Work out the finished part from the listing and answer in its coordinate system (mm). A direction names the side the tool comes from. Give positions to 0.01 mm unless a question says otherwise; leave off trailing zeros. Order: outer loops, then holes, each group sorted by start corner. A loop starts at its lowest first (then second) coordinate and runs counter-clockwise, first axis right, second up.
```python
from build123d import *

# Parameters (mm, degrees)
F1_DEPTH = 787.4
F3_DEPTH = 25.4
F4_SIZE  = 5.08


with BuildPart() as f1:
    # F0 (on Right) → F1 (new body)
    with BuildSketch(Plane.YZ):
        with BuildLine():
            Line((-17.145, 0), (0, 0))
            Line((0, 0), (0, 101.6))
            Line((0, 101.6), (-12.7, 101.6))
            Line((-12.7, 101.6), (-12.7, 98.425))
            ThreePointArc((-12.7, 98.425), (-21.680256, 94.705256), (-25.4, 85.725))
            Line((-25.4, 85.725), (-25.4, 38.1))
            Line((-25.4, 38.1), (-17.145, 38.1))
            Line((-17.145, 38.1), (-17.145, 0))
        make_face()
    extrude(amount=F1_DEPTH)

    # F2 (on face) → F3 (cut)
    with BuildSketch(Plane(origin=(0, 0, 0), x_dir=(-1, 0, 0), z_dir=(0, 1, 0))):
        Polygon((-685.8, 0), (-787.4, 101.6), (-787.4, 0), align=None)
        Polygon((0, 0), (0, 101.6), (-101.6, 0), align=None)
    extrude(amount=-F3_DEPTH, mode=Mode.SUBTRACT)

    # F4
    f4_edges = [f1.edges().sort_by_distance(p)[0] for p in [
        (393.7, -25.4, 38.1),
    ]]
    chamfer(f4_edges, length=F4_SIZE)


solid = f1.part
```
1. Which of the six approach directions +Z, -Z, +X, -X, +Y, -Y give full straight-line access (tool end or side, diameter ignored) to faces 1 (the face through (389, -17.145, 19)), 2 (the face through (50.1, -9.7, 51.5))?
Findings below:
face 1: -Z, +X, -X, -Y
face 2: -Z, -X, +Y, -Y
2. Given P1, Ø2.5, axis at x = 483.5, z = 100.5, coming from the -Y side; P2, Ø1, axis at x = 105, z = 31, coming from the -Y side (3 decimals); P3, Ø1.5, axis at x = 521, y = -22, coming from the -Z side, each flat-ended and moving along its own axis, determine where each tip first touches the part or whether it passes through.
Findings below:
P1: stops at y = -12.7
P2: stops at y = -17.145
P3: stops at z = 39.03
3. The part is cut by section A-A (x = 218). Write down the section's boundary in (y, z) (3 decimals), then the cut area to 3 significant figures.
Findings below:
outline: (-25.4, 43.18) - (-20.32, 38.1) - (-17.145, 38.1) - (-17.145, 0) - (0, 0) - (0, 101.6) - (-12.7, 101.6) - (-12.7, 98.425) arc R12.7 ccw to (-25.4, 85.725) - close
area: 2,180 mm2
4. The part is cut by section D-D (x = 700). Write down the section's boundary in (y, z) (3 decimals).
Findings below:
outline: (-25.4, 43.18) - (-20.32, 38.1) - (-17.145, 38.1) - (-17.145, 14.2) - (0, 14.2) - (0, 101.6) - (-12.7, 101.6) - (-12.7, 98.425) arc R12.7 ccw to (-25.4, 85.725) - close
5. The mould has two halves that part along Y. Classify faces 3 (the face through (388, -6, 101.6)), 4 (the face through (388, 0, 50)), 5 (the face through (388.233, -21.581, 94.803)): pulls with the +Y half, pulls with the -Y half, needs draft (parallel to the pull), parting line crosses it, or undercut.
Findings below:
face 3: needs draft
face 4: pulls with the +Y half
face 5: pulls with the -Y half
6. Straight lines are drawn through the part: probe 1 along Y at (x, z) = (241.5, 35.5) (3 decimals); probe 2 along X at (y, z) = (-7, 5); probe 3 along X at (y, z) = (-9.5, 91.5). For each, find the intervals that lie inside material, in ascending order.
Findings below:
probe 1: y = -17.145 to 0
probe 2: x = 96.6 to 690.8
probe 3: x = 10.1 to 777.3
7. The part is cut by section B-B (z = 56.5). Write down the section's boundary in (x, y).
Findings below:
outline: (45.1, -25.4) - (742.3, -25.4) - (742.3, 0) - (45.1, 0) - close
8. The part is cut by section C-C (y = -4.25). Write down the section's boundary in (x, z).
Findings below:
outline: (0, 101.6) - (101.6, 0) - (685.8, 0) - (787.4, 101.6) - close
